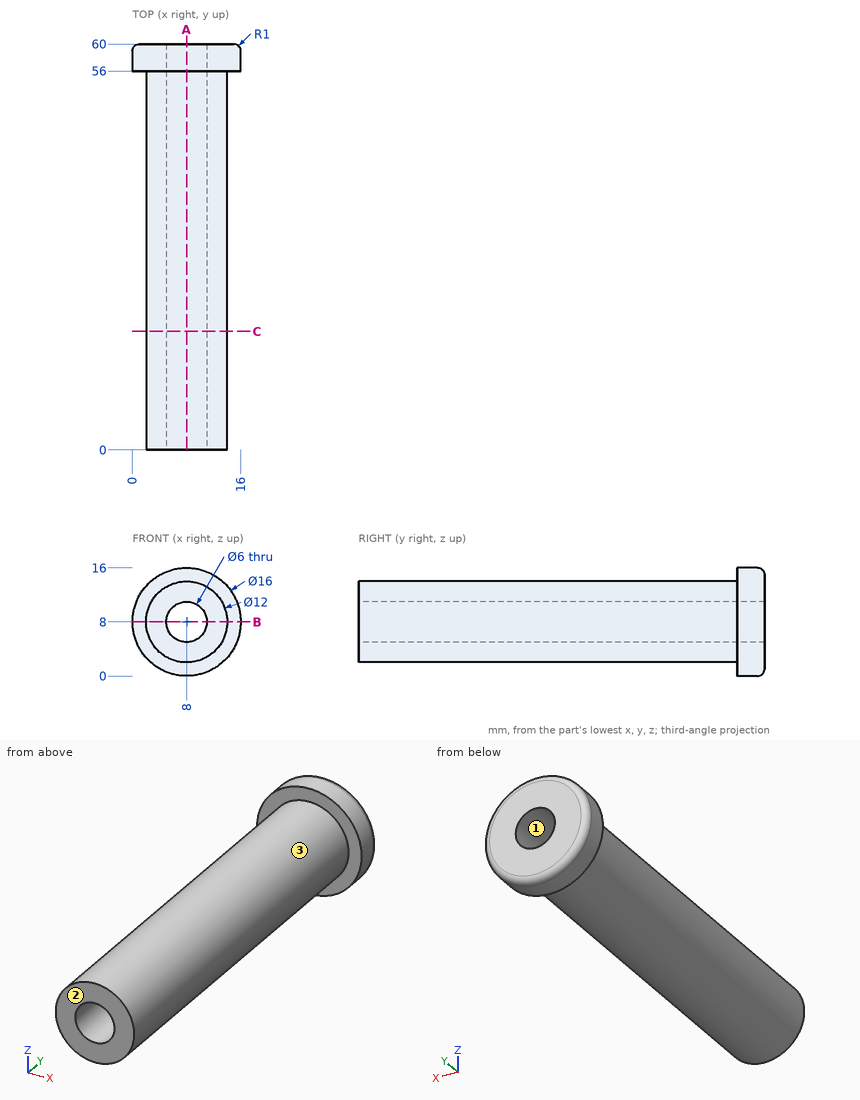
Drawing for the job (mm, zero at the part's lowest x, y, z). Round coordinates to 2 decimals unless told otherwise and drop trailing zeros. Order: outer loops, then holes, each group sorted by start corner. A loop starts at its lowest first (then second) coordinate and runs counter-clockwise, first axis right, second up.
Item 1: Saw through at A-A on x = 8. Write the cut outline in (y, z), then the cut area to 3 significant figures.
Item 2: Probe line 1 along Z through (x, y) = (8, 30); line 2 along X through (y, z) = (42, 7.75); line 3 along Y through (x, z) = (1.5, 7.75). List the from-to ranges inside material, lowest first.
Item 3: Saw through at C-C on y = 17.5. Write the cut outline in (x, z), then the cut area to 3 significant figures.
Item 4: Pin check, flat tips, straight feed: pin 1 (8 mm diameter, centred on y = 36.5, z = 9, fed in from +X); pin 2 (1.5 mm diameter, centred on y = 44, z = 13.5, fed in from +X); pin 3 (5.5 mm diameter, centred on x = 8, z = 8, fed in from +Y); pin 4 (1.5 mm diameter, centred on x = 12, y = 28.5, fed in from +Z). Stop position of each tip, or through.
Item 5: Saw through at B-B on z = 8. Write the cut outline in (x, y).
Item 6: Mould opens along X. For the marked faces 1, 2 and 3 say: pulls with the +X half, pulls with the -X half, needs draft (parallel to the pull), parting line crosses it, or undercut.
Reported:
1. outline: (0, 2) - (56, 2) - (56, 0) - (59, 0) arc R1 ccw to (60, 1) - (60, 5) - (0, 5) - close; (0, 11) - (60, 11) - (60, 15) arc R1 ccw to (59, 16) - (56, 16) - (56, 14) - (0, 14) - close
1. area: 376 mm2
2. line 1: z = 2 to 5, 11 to 14
2. line 2: x = 2.01 to 5.01, 10.99 to 13.99
2. line 3: y = 56 to 60
3. outline: circle Ø12 at (8, 8); hole circle Ø6 at (8, 8)
3. area: 84.8 mm2
4. pin 1: stops at x = 14
4. pin 2: stops at x = 11.67
4. pin 3: passes through
4. pin 4: stops at z = 13.04
5. outline: (0, 56) - (2, 56) - (2, 0) - (5, 0) - (5, 60) - (1, 60) arc R1 ccw to (0, 59) - close; (11, 0) - (14, 0) - (14, 56) - (16, 56) - (16, 59) arc R1 ccw to (15, 60) - (11, 60) - close
6. face 1: undercut
6. face 2: needs draft
6. face 3: parting line crosses it
